Read the model definition and answer for the solid it produces. Units are mm, in the model's axes. A direction names the side the tool comes from. Coordinates: 2 decimals unless noted, no trailing zeros. Write each loop counter-clockwise with the first axis right and the second up, starting at its lowest first coordinate (ties: lowest second). Pieces come first, ordered by that corner, then holes. Notation, with made-up numbers: (-12, 66.5) -> (24, 66.5) arc R13 ccw to (24, 89.5) -> close; hole circle Ø8 at (-9.5, 15). An arc over 180 degrees is marked (long way). Answer in a Markdown table with one row per item. Add a question column.
Item 1: Which of the six approach directions +Z, -Z, +X, -X, +Y, -Y give full straight-line access (tool end or side, diameter ignored) to faces 1 (the face through (-26.6, 8, -7)), 2 (the face through (0, 7, 14.25)), 3 (the face through (28.4, 1.4, -1.2))?
Item 2: Section B-B on x = -16.35 is taken. Write down the section's boundary in (y, z), then the cut area to 3 significant figures.
Item 3: Given pin 1 Ø2 at (y, z) = (2.5, -2) entering from +X; pin 2 Ø1.8 at (y, z) = (2, 2) entering from +X; pin 3 Ø10 at (x, z) = (8, -1.5) entering from +Y; pin 4 Ø1.1 at (x, y) = (-16.5, 14.5) entering from +Z, each flat-ended and moving along its own axis, determine where each tip first touches the part or whether it passes through.
Item 4: Section A-A on z = 0 is taken. Write down the section's boundary in (x, y).
Item 5: For a pull along Y with two mould halves and no side action, classify faces 4 (the face through (-28, 15, 0)), 5 (the face through (17.53, 12.48, -13.39)), 6 (the face through (-22.6, 13.5, 13)) as +Y half, -Y half, draft (parallel to the pull), parting line (faces both ways), or undercut.
Item 6: Section D-D on x = -4.5 is taken. Write down the section's boundary in (y, z), then the cut area to 3 significant figures.
Item 7: Straight lines are drawn through the part: line 1 (X direction, y = 0.75, z = 0); line 2 (X direction, y = 8.5, z = 11.5); line 3 (Z direction, x = 16.35, y = 0.35). For each, find the intervals that lie inside material, in ascending order. Write a range as from..to.
Item 8: Section C-C on y = 2 is taken. Write down the section's boundary in (x, z).
Autodesk Inventor part; units mm, degrees
ref_plane "YZ Plane" through (0, 0, 0) normal (1, 0, 0) x (0, 1, 0)
ref_plane "XZ Plane" through (0, 0, 0) normal (0, 1, 0) x (-1, 0, 0)
ref_plane "XY Plane" through (0, 0, 0) normal (0, 0, 1) x (1, 0, 0)
sketch "Sketch1" plane through (0, 0, 0) normal (1, 0, 0) x (0, 1, 0)
  line L0 (15, 15.25) -> (0, 15.25)
  line L1 (0, 15.25) -> (0, -15.25)
  line L2 (0, -15.25) -> (15, -15.25)
  line L3 (15, -15.25) -> (15, 15.25)
  line L4 (15, 15.25) -> (0, -15.25) construction
  line L5 (0, 15.25) -> (15, -15.25) construction
  point P0 (0, 0)
  point P1 (7.5, 0)
  dimension "d0" = 15
  dimension "d1" = 30.5
  dimension "d2" = 0
  dimension "d3" = 0
extrude "Extrusion1" add sketch "Sketch1" along normal mid plane 57.2
fillet "Fillet1" radius 5 2 edges at (0, 15, 15.25) (0, 15, -15.25)
sketch "Sketch2" plane through (0, 0, 0) normal (1, 0, 0) x (0, 1, 0)
  arc A0 (10, -15.25) -> (15, -10.25) centre (10, -10.25) ccw
  line L0 (15, -10.25) -> (15, 10.25)
  arc A1 (15, 10.25) -> (10, 15.25) centre (10, 10.25) ccw
  line L1 (10, 15.25) -> (0, 15.25)
  line L2 (0, 15.25) -> (0, -15.25)
  line L3 (0, -15.25) -> (10, -15.25)
  line L4 (1, 14.25) -> (10, 14.25)
  arc A2 (14, 10.25) -> (10, 14.25) centre (10, 10.25) ccw
  line L5 (14, 10.25) -> (14, -10.25)
  arc A3 (10, -14.25) -> (14, -10.25) centre (10, -10.25) ccw
  line L6 (10, -14.25) -> (1, -14.25)
  line L7 (1, -14.25) -> (1, 14.25)
  point P0 (0, 0)
  dimension "d7" = 1
extrude "Extrusion2" cut sketch "Sketch2" along normal mid plane 55.2 contours L4 A2 L5 A3 L6 L7
sketch "Sketch3" plane through (-28.6, 15, -10.25) normal (0, 1, 0) x (1, 0, 0)
  line L0 (0, -20.5) -> (0, 0) construction
  line L1 (57.2, -20.5) -> (0, -20.5) construction
  line L2 (57.2, 0) -> (57.2, -20.5) construction
  line L3 (1, 4) -> (1, -24.5)
  line L4 (1, -24.5) -> (6, -24.5)
  line L5 (6, -24.5) -> (6, -21.5)
  line L6 (6, -21.5) -> (16, -21.5)
  line L7 (16, -21.5) -> (16, -24.5)
  line L8 (16, -24.5) -> (41.2, -24.5)
  line L9 (41.2, -24.5) -> (41.2, -21.5)
  line L10 (41.2, -21.5) -> (51.2, -21.5)
  line L11 (51.2, -21.5) -> (51.2, -24.5)
  line L12 (51.2, -24.5) -> (56.2, -24.5)
  line L13 (56.2, -24.5) -> (56.2, 4)
  line L14 (56.2, 4) -> (51.2, 4)
  line L15 (51.2, 4) -> (51.2, 1)
  line L16 (51.2, 1) -> (41.2, 1)
  line L17 (41.2, 1) -> (41.2, 4)
  line L18 (41.2, 4) -> (16, 4)
  line L19 (16, 4) -> (16, 1)
  line L20 (16, 1) -> (6, 1)
  line L21 (6, 1) -> (6, 4)
  line L22 (6, 4) -> (1, 4)
  line L23 (57.2, 5) -> (0, 5)
  line L24 (0, -25.5) -> (57.2, -25.5)
  point P0 (28.6, -10.25)
  dimension "d10" = 1
  dimension "d11" = 1
  dimension "d12" = 1
  dimension "d13" = 1
  dimension "d14" = 10
  dimension "d15" = 5
  dimension "d16" = 3
extrude "Extrusion3" cut sketch "Sketch3" against normal up to next
sketch "Sketch4" plane through (-27.6, 1, 14.25) normal (0, 1, 0) x (1, 0, 0)
  line L0 (0, 0) -> (55.2, 0)
  line L1 (55.2, 28.5) -> (0, 28.5)
  point P0 (27.6, 14.25)
  point P1 (11.25, 14.25)
  point P2 (43.95, 14.25)
  dimension "d19" = 32.7
  dimension "d20" = 16.35
  dimension "d21" = 14.25
  dimension "d22" = 14.25
  dimension "d23" = 14.25
hole "Hole1" at (-16.35, 1, 0) at (16.35, 1, 0) direction (0, -1, 0) diameter 2.7 end through all
sketch "Sketch5" plane through (-27.6, 0, 0) normal (1, 0, 0) x (0, 0, -1)
  line L0 (14.25, 1) -> (-14.25, 1)
  line L1 (-10.25, 15) -> (10.25, 15)
  circle A0 centre (7.2, 8.2) radius 1.2755
  line L2 (0, 0) -> (0, 12.8621) construction
  dimension "d31" = 7.2
  dimension "d32" = 7.2
extrude "Extrusion4" add sketch "Sketch5" along normal blind 1
pattern_circular "Circular Pattern1" count 2 over 360 about axis through (0, -10, 0) along (0, 1, 0) of "Extrusion4"
sketch "Sketch6" plane through (28.6, 0, 0) normal (1, 0, 0) x (0, 0, -1)
  circle A0 centre (-2, 2) radius 1
  circle A1 centre (2, 2) radius 1
  line L0 (-14.25, 1) -> (14.25, 1)
  point P0 (0, 0)
  dimension "d38" = 2
  dimension "d39" = 2
  dimension "d40" = 2
  dimension "d41" = 2
extrude "Extrusion5" cut sketch "Sketch6" against normal blind 0.5
sketch "Sketch7" plane through (28.6, 0, 0) normal (1, 0, 0) x (0, 0, -1)
  circle A0 centre (2, 2) radius 1
sketch "Sketch8" plane through (28.6, 0, 0) normal (1, 0, 0) x (0, 0, -1)
  circle A0 centre (-2, 2) radius 1
equation "\"d13\" = d12"
equation "\"d32\" = d31"
properties part number "AAHolder" material "ABS Plastic"
Results below:
| question | item | result |
|---|---|---|
| 1 | face 1 | +Y |
| 1 | face 2 | none |
| 1 | face 3 | +X |
| 2 | outline | (0, -15.25) -> (10, -15.25) arc R5 ccw to (14.9, -11.25) -> (13.87, -11.25) arc R4 cw to (10, -14.25) -> (1, -14.25) -> (1, -1.35) -> (0, -1.35) -> close; (0, 1.35) -> (1, 1.35) -> (1, 14.25) -> (10, 14.25) arc R4 cw to (13.87, 11.25) -> (14.9, 11.25) arc R5 ccw to (10, 15.25) -> (0, 15.25) -> close |
| 2 | area | 57.9 mm2 |
| 3 | pin 1 | stops at x = 28.6 |
| 3 | pin 2 | stops at x = 28.1 |
| 3 | pin 3 | stops at y = 1 |
| 3 | pin 4 | stops at z = 13.32 |
| 4 | outline | (-28.6, 0) -> (-17.7, 0) -> (-17.7, 1) -> (-27.6, 1) -> (-27.6, 15) -> (-28.6, 15) -> close; (-15, 0) -> (15, 0) -> (15, 1) -> (-15, 1) -> close; (17.7, 0) -> (28.6, 0) -> (28.6, 15) -> (27.6, 15) -> (27.6, 1) -> (17.7, 1) -> close |
| 5 | face 4 | +Y half |
| 5 | face 5 | undercut |
| 5 | face 6 | draft |
| 6 | outline | (0, -15.25) -> (10, -15.25) arc R5 ccw to (13, -14.25) -> (1, -14.25) -> (1, 14.25) -> (13, 14.25) arc R5 ccw to (10, 15.25) -> (0, 15.25) -> close |
| 6 | area | 52.6 mm2 |
| 7 | line 1 | x = -28.6..-17.7, -15..15, 17.7..28.6 |
| 7 | line 2 | x = -28.6..-27.6, 27.6..28.6 |
| 7 | line 3 | z = -15.25..-1.35, 1.35..15.25 |
| 8 | outline | (-28.6, -15.25) -> (28.6, -15.25) -> (28.6, -3) -> (28.1, -3) -> (28.1, -1) -> (28.6, -1) -> (28.6, 1) -> (28.1, 1) -> (28.1, 3) -> (28.6, 3) -> (28.6, 15.25) -> (-28.6, 15.25) -> close; hole (-27.6, -14.25) -> (27.6, -14.25) -> (27.6, 14.25) -> (-27.6, 14.25) -> close |
